Read the model definition and answer for the solid it produces. Units are mm, in the model's axes. A direction names the side the tool comes from. Give positions to 0.01 mm unless a question says otherwise; leave off trailing zeros. Write each loop counter-clockwise with the first axis right and the second up, starting at its lowest first coordinate (ties: lowest second). Pieces come first, ordered by that corner, then holes. Notation, with made-up numbers: M -34.5,-3.75 L 17.5,-3.75 A29 ccw 17.5,33.25 Z; hole C -2.75,-17 d11. An arc over 180 degrees is marked long. Use a Markdown table: item, result. Add a question column.
Item 1: A cutting plane is placed at A-A on x = -25. Determine the outline of the cut face in (y, z).
Item 2: A cutting plane is placed at D-D on z = 99.5. Count the separate pieces of the cut face and the enclosed holes in it, then the cut area to 3 significant figures.
Item 3: The mould has two halves that part along X. Classify faces 5 (the flat face through (24, 30, 69)), 6 (the flat face through (-7, -25, 57)), 7 (the flat face through (-30, 24, 67)): pulls with the +X half, pulls with the -X half, needs draft (parallel to the pull), parting line crosses it, or undercut.
Item 4: A cutting plane is placed at C-C on x = 14. Determine the outline of the cut face in (y, z).
Item 5: Given P1, Ø8, axis at x = -18, y = -13.5, coming from the -Z side; P2, Ø1.3, axis at y = 13, z = 85, coming from the +X side; P3, Ø3, axis at y = -14, z = 50.5, coming from the +X side, each flat-ended and moving along its own axis, determine where each tip first touches the part or whether it passes through.
Item 6: A cutting plane is placed at B-B on y = -5. Determine the outline of the cut face in (x, z), then the cut area to 3 significant figures.
Item 7: Consider probe 1 along Y at (x, z) = (15, 52.5); probe 2 along Y at (x, z) = (25, 92). Determine where each line is inside the solid, lowest interval first. Write a range as [from, to].
Item 8: For faces 1 (the flat face through (18.15, 29, 69)), 2 (the flat face through (20.15, -24, 57)), 3 (the flat face through (29, 11.85, 66)), 4 (the flat face through (-11.85, -29, 57)), determine the directions among +Z, -Z, +X, -X, +Y, -Y from which every point of the face is accessible in a straight line to the end or side of a thin tool.
from build123d import *

# Parameters (mm, degrees)
F0_R          = 3
F0_R_2        = 2.5
F1_DEPTH      = 140
F2_R          = 2
F3_R          = 7
F6_DEPTH      = 30
F6_DEPTH_BACK = 30
F7_W          = 131.1645284295
F7_H          = 50.7057756186
F8_DEPTH      = 30
F8_DEPTH_BACK = 30


# Not quite as in the source:
# - a feature names something its author has since deleted; it is built from what else it names


with BuildPart() as f1:
    # F0 (on Top) → F1 (new body)
    with BuildSketch(Plane.XY):
        with BuildLine():
            Line((18.15, -30), (30, -30))
            Line((30, -30), (30, -18.15))
            Line((30, -18.15), (27.5, -18.15))
            Line((27.5, -18.15), (27.5, -20.15))
            Line((27.5, -20.15), (21.5477069044, -20.15))
            ThreePointArc((21.5477069044, -20.15), (19.5, -15), (21.5477069044, -9.85))
            Line((21.5477069044, -9.85), (27.5, -9.85))
            Line((27.5, -9.85), (27.5, -11.85))
            Line((27.5, -11.85), (30, -11.85))
            Line((30, -11.85), (30, 11.85))
            Line((30, 11.85), (27.5, 11.85))
            Line((27.5, 11.85), (27.5, 9.85))
            Line((27.5, 9.85), (21.5477069044, 9.85))
            ThreePointArc((21.5477069044, 9.85), (19.5, 15), (21.5477069044, 20.15))
            Line((21.5477069044, 20.15), (27.5, 20.15))
            Line((27.5, 20.15), (27.5, 18.15))
            Line((27.5, 18.15), (30, 18.15))
            Line((30, 18.15), (30, 30))
            Line((30, 30), (18.15, 30))
            Line((18.15, 30), (18.15, 27.5))
            Line((18.15, 27.5), (20.15, 27.5))
            Line((20.15, 27.5), (20.15, 21.5477069044))
            ThreePointArc((20.15, 21.5477069044), (15, 19.5), (9.85, 21.5477069044))
            Line((9.85, 21.5477069044), (9.85, 27.5))
            Line((9.85, 27.5), (11.85, 27.5))
            Line((11.85, 27.5), (11.85, 30))
            Line((11.85, 30), (-11.85, 30))
            Line((-11.85, 30), (-11.85, 27.5))
            Line((-11.85, 27.5), (-9.85, 27.5))
            Line((-9.85, 27.5), (-9.85, 21.5477069044))
            ThreePointArc((-9.85, 21.5477069044), (-15, 19.5), (-20.15, 21.5477069044))
            Line((-20.15, 21.5477069044), (-20.15, 27.5))
            Line((-20.15, 27.5), (-18.15, 27.5))
            Line((-18.15, 27.5), (-18.15, 30))
            Line((-18.15, 30), (-30, 30))
            Line((-30, 30), (-30, 18.15))
            Line((-30, 18.15), (-27.5, 18.15))
            Line((-27.5, 18.15), (-27.5, 20.15))
            Line((-27.5, 20.15), (-21.5477069044, 20.15))
            ThreePointArc((-21.5477069044, 20.15), (-19.5, 15), (-21.5477069044, 9.85))
            Line((-21.5477069044, 9.85), (-27.5, 9.85))
            Line((-27.5, 9.85), (-27.5, 11.85))
            Line((-27.5, 11.85), (-30, 11.85))
            Line((-30, 11.85), (-30, -11.85))
            Line((-30, -11.85), (-27.5, -11.85))
            Line((-27.5, -11.85), (-27.5, -9.85))
            Line((-27.5, -9.85), (-21.5477069044, -9.85))
            ThreePointArc((-21.5477069044, -9.85), (-19.5, -15), (-21.5477069044, -20.15))
            Line((-21.5477069044, -20.15), (-27.5, -20.15))
            Line((-27.5, -20.15), (-27.5, -18.15))
            Line((-27.5, -18.15), (-30, -18.15))
            Line((-30, -18.15), (-30, -30))
            Line((-30, -30), (-18.15, -30))
            Line((-18.15, -30), (-18.15, -27.5))
            Line((-18.15, -27.5), (-20.15, -27.5))
            Line((-20.15, -27.5), (-20.15, -21.5477069044))
            ThreePointArc((-20.15, -21.5477069044), (-15, -19.5), (-9.85, -21.5477069044))
            Line((-9.85, -21.5477069044), (-9.85, -27.5))
            Line((-9.85, -27.5), (-11.85, -27.5))
            Line((-11.85, -27.5), (-11.85, -30))
            Line((-11.85, -30), (11.85, -30))
            Line((11.85, -30), (11.85, -27.5))
            Line((11.85, -27.5), (9.85, -27.5))
            Line((9.85, -27.5), (9.85, -21.5477069044))
            ThreePointArc((9.85, -21.5477069044), (15, -19.5), (20.15, -21.5477069044))
            Line((20.15, -21.5477069044), (20.15, -27.5))
            Line((20.15, -27.5), (18.15, -27.5))
            Line((18.15, -27.5), (18.15, -30))
        make_face()
        with Locations((-25, -25)):
            Circle(F0_R, mode=Mode.SUBTRACT)
        with Locations((-15, -15)):
            Circle(F0_R_2, mode=Mode.SUBTRACT)
        with Locations((25, -25)):
            Circle(F0_R, mode=Mode.SUBTRACT)
        with Locations((15, -15)):
            Circle(F0_R_2, mode=Mode.SUBTRACT)
        with Locations((-25, 25)):
            Circle(F0_R, mode=Mode.SUBTRACT)
        with Locations((-15, 15)):
            Circle(F0_R_2, mode=Mode.SUBTRACT)
        Polygon((-7, 22), (-7, 27.5), (0, 27.5), (7, 27.5), (7, 22), (10, 16), (10, 10), (16, 10), (22, 7), (27.5, 7), (27.5, 0), (27.5, -7), (22, -7), (16, -10), (10, -10), (10, -16), (7, -22), (7, -27.5), (0, -27.5), (-7, -27.5), (-7, -22), (-10, -16), (-10, -10), (-16, -10), (-22, -7), (-27.5, -7), (-27.5, 0), (-27.5, 7), (-22, 7), (-16, 10), (-10, 10), (-10, 16), align=None, mode=Mode.SUBTRACT)
        with Locations((15, 15)):
            Circle(F0_R_2, mode=Mode.SUBTRACT)
        with Locations((25, 25)):
            Circle(F0_R, mode=Mode.SUBTRACT)
    extrude(amount=F1_DEPTH)

    # F2
    f2_edges = [f1.edges().sort_by_distance(p)[0] for p in [
        (-7, 27.5, 70),
        (7, 27.5, 70),
    ]]
    fillet(f2_edges, radius=F2_R)

    # F3
    f3_edges = [f1.edges().sort_by_distance(p)[0] for p in [
        (-10, 16, 70),
        (10, 16, 70),
    ]]
    fillet(f3_edges, radius=F3_R)

    # F5 (on Right) → F6 (cut, two sides)
    with BuildSketch(Plane.YZ) as f6_sk:
        Polygon((214.5999793503, -135.2321386172), (130.9673605882, 66.674863855), (-30, 0), (53.6326187621, -201.9070024722), align=None)
        Polygon((30, 140), (-2.0081647111, 217.2745453523), (-162.3392477394, 150.863236292), (-130.3310830283, 73.5886909397), align=None)
    extrude(amount=-F6_DEPTH, mode=Mode.SUBTRACT)
    extrude(f6_sk.sketch, amount=F6_DEPTH_BACK, mode=Mode.SUBTRACT)

    # F7 (on Right) → F8 (cut, two sides)
    with BuildSketch(Plane.YZ) as f8_sk:
        with Locations((35.5822642148, 140.5000740669)):
            Rectangle(F7_W, F7_H)
    extrude(amount=F8_DEPTH, mode=Mode.SUBTRACT)
    extrude(f8_sk.sketch, amount=-F8_DEPTH_BACK, mode=Mode.SUBTRACT)


solid = f1.part
Filled in:
| question | item | result |
|---|---|---|
| 1 | outline | M -30,0 L -28,0.83 L -28,115.15 L -30,115.15 Z; M -22,3.31 L -20.15,4.08 L -20.15,115.15 L -22,115.15 Z; M -9.85,8.35 L -7,9.53 L -7,115.15 L -9.85,115.15 Z; M 7,15.33 L 9.85,16.51 L 9.85,115.15 L 7,115.15 Z; M 20.15,20.77 L 22,21.54 L 22,115.15 L 20.15,115.15 Z; M 28,24.02 L 30,24.85 L 30,115.15 L 28,115.15 Z |
| 2 | separate pieces | 1 |
| 2 | enclosed holes | 9 |
| 2 | area | 1,080 mm² |
| 3 | face 5 | needs draft |
| 3 | face 6 | undercut |
| 3 | face 7 | pulls with the -X half |
| 4 | outline | M -19.57,4.32 L -17.29,5.26 L -17.29,115.15 L -19.57,115.15 Z; M -12.71,7.16 L -10,8.28 L -10,115.15 L -12.71,115.15 Z; M 10,16.57 L 12.71,17.69 L 12.71,115.15 L 10,115.15 Z; M 17.29,19.59 L 19.57,20.53 L 19.57,115.15 L 17.29,115.15 Z |
| 5 | P1 | z = 5.18 |
| 5 | P2 | x = 19.98 |
| 5 | P3 | x = 19.93 |
| 6 | outline | M -30,10.36 L -27.5,10.36 L -27.5,115.15 L -30,115.15 Z; M 27.5,10.36 L 30,10.36 L 30,115.15 L 27.5,115.15 Z |
| 6 | area | 524 mm² |
| 7 | probe 1 | [-19.5, -17.5], [-12.5, -10], [10, 12.5], [17.5, 19.5] |
| 7 | probe 2 | [-30, -28], [-22, -20.15], [-9.85, -7], [7, 9.85], [20.15, 22], [28, 30] |
| 8 | face 1 | +Z, -Z, +Y |
| 8 | face 2 | +Z, -Z |
| 8 | face 3 | +Z, -Z, +X |
| 8 | face 4 | +Z, -Z, -Y |
